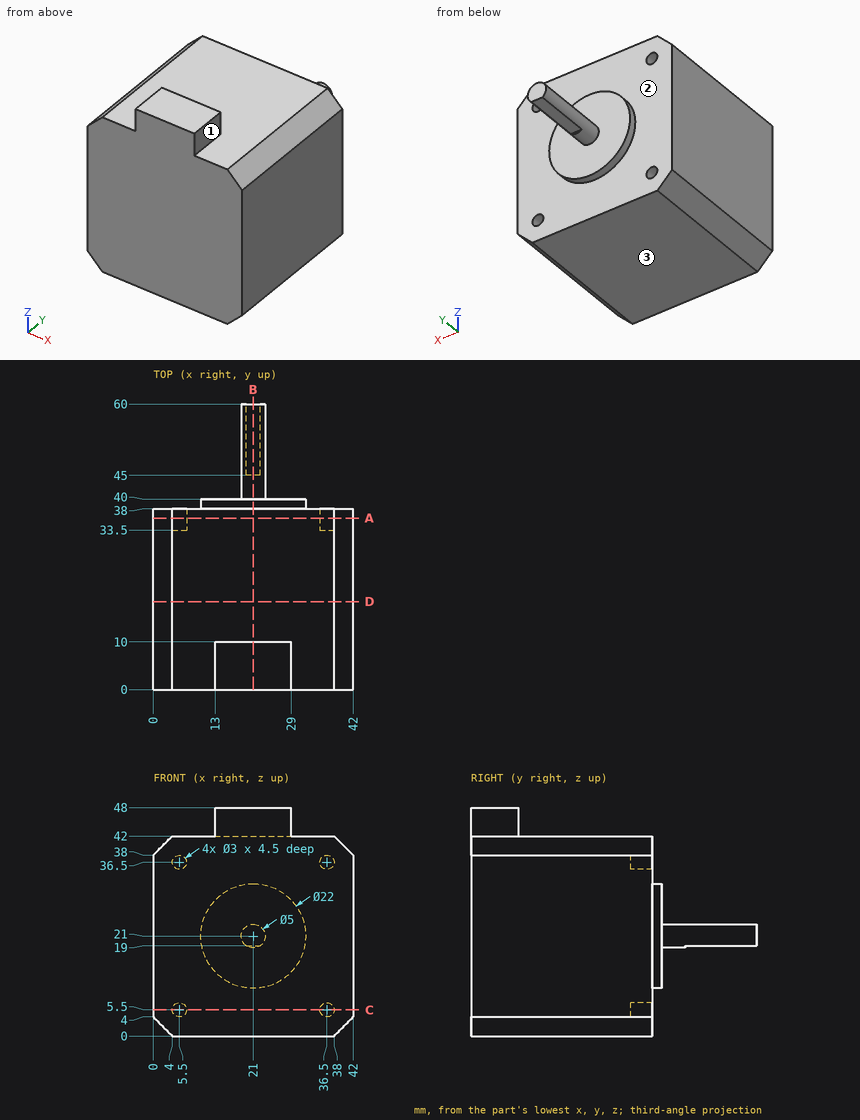
Could you check a few things on this drawing? It's one solid part, dimensions in mm from its lowest x, y, z. A direction names the side the tool comes from. Round coordinates to 2 decimals unless told otherwise and drop trailing zeros. Write each loop counter-clockwise with the first axis right and the second up, starting at its lowest first coordinate (ties: lowest second). Pieces come first, ordered by that corner, then holes. Notation, with made-up numbers: M -27,-14 L 31,-14 A26 ccw 31,10 Z; hole C 3,-28.5 d11. An arc over 180 degrees is marked long. Answer as CSV lines item,"result". Start each with the question number.
1. On a 3-axis mill with a long thin cutter (end or side, diameter ignored), from which of +Z, -Z, +X, -X, +Y, -Y can I reach the whole of each face in a straight line? I mean the marked faces 1, 2 and 3. Say none if no direction works.
2. Suppose I cut it at B-B on x = 21. Write out the boundary of the cut face in (y, z).
3. I'm going to push flat-ended pins straight in: pin 1 Ø0.9 at (x, z) = (36, 37) entering from +Y; pin 2 Ø6.5 at (x, z) = (23.5, 26) entering from +Y; pin 3 Ø4 at (x, z) = (5.5, 36.5) entering from +Y; pin 4 Ø3.5 at (x, y) = (21.5, 54.5) entering from -Z. Where does each tip first touch, or does it pass through?
4. Suppose I cut it at D-D on y = 18.5. Write out the boundary of the cut face in (x, z).
5. I need wall thicknesses on probe 1 along X at (y, z) = (35.8, 5.5); probe 2 along Y at (x, z) = (35, 40). Which ranges of each line are inside material? Lowest first, please.
6. Suppose I cut it at A-A on y = 36. Write out the boundary of the cut face in (x, z), then the cut area to 3 significant figures.
7. Suppose I cut it at C-C on z = 5.5. Write out the boundary of the cut face in (x, y), then the cut area to 3 significant figures.
Check result:
1,face 1,"+Z, +X, +Y, -Y"
1,face 2,"+Y"
1,face 3,"-Z, +X, -X, +Y, -Y"
2,outline,"M 0,0 L 38,0 L 38,10 L 40,10 L 40,18.5 L 45,18.5 L 45,19 L 60,19 L 60,23.5 L 40,23.5 L 40,32 L 38,32 L 38,42 L 10,42 L 10,48 L 0,48 Z"
3,pin 1,"stops at y = 33.5"
3,pin 2,"stops at y = 60"
3,pin 3,"stops at y = 38"
3,pin 4,"stops at z = 19"
4,outline,"M 0,4 L 4,0 L 38,0 L 42,4 L 42,38 L 38,42 L 4,42 L 0,38 Z"
5,probe 1,"x = 0 to 4, 7 to 35, 38 to 42"
5,probe 2,"y = 0 to 38"
6,outline,"M 0,4 L 4,0 L 38,0 L 42,4 L 42,38 L 38,42 L 4,42 L 0,38 Z; hole C 5.5,5.5 d3; hole C 5.5,36.5 d3; hole C 36.5,5.5 d3; hole C 36.5,36.5 d3"
6,area,"1,700 mm2"
7,outline,"M 0,0 L 42,0 L 42,38 L 38,38 L 38,33.5 L 35,33.5 L 35,38 L 7,38 L 7,33.5 L 4,33.5 L 4,38 L 0,38 Z"
7,area,"1,570 mm2"
